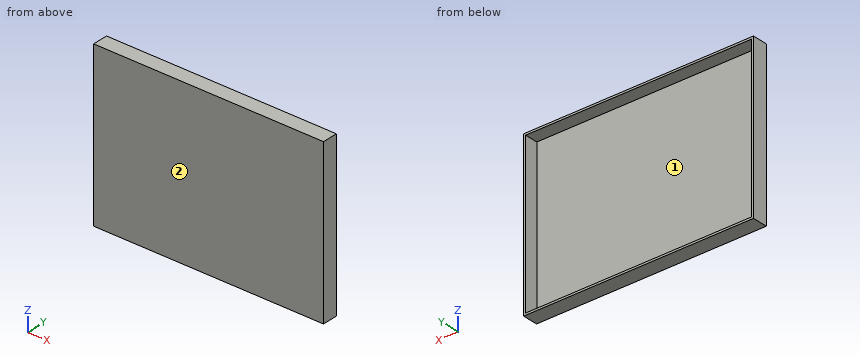
```python
from build123d import *

# Parameters (mm, degrees)
SKETCH1_W           = 343
SKETCH1_H           = 243
SKETCH1_W_2         = 337
SKETCH1_H_2         = 237
BOSS_EXTRUDE1_DEPTH = 23
SKETCH2_W           = 343
SKETCH2_H           = 243
BOSS_EXTRUDE2_DEPTH = 3


with BuildPart() as part:
    # Sketch1 → Boss-Extrude1 (new body)
    with BuildSketch(Plane(origin=(0, 0, 0), x_dir=(1, 0, 0), z_dir=(0, 1, 0))):
        Rectangle(SKETCH1_W, SKETCH1_H)
        Rectangle(SKETCH1_W_2, SKETCH1_H_2, mode=Mode.SUBTRACT)
    extrude(amount=BOSS_EXTRUDE1_DEPTH)

    # Sketch2 → Boss-Extrude2 (add)
    with BuildSketch(Plane.XZ):
        Rectangle(SKETCH2_W, SKETCH2_H)
    extrude(amount=-BOSS_EXTRUDE2_DEPTH)


solid = part.part
```
For this review, take the finished solid that the model builds, in its own axes (mm). Face numbers are marked on the shaded views. Round coordinates to 2 decimals unless told otherwise and drop trailing zeros. Write each loop counter-clockwise with the first axis right and the second up, starting at its lowest first coordinate (ties: lowest second). Pieces come first, ordered by that corner, then holes. Notation, with made-up numbers: (47.25, 3.5) - (71.25, 3.5) arc R37 ccw to (71.25, 39.5) - close; hole circle Ø9 at (83, 62.5). An arc over 180 degrees is marked (long way). Put each result on its own line as item: value.
Q1. We need section C-C (x = 134). Give the boundary of the cut face in (y, z).
Solved:
outline: (0, -121.5) - (23, -121.5) - (23, -118.5) - (3, -118.5) - (3, 118.5) - (23, 118.5) - (23, 121.5) - (0, 121.5) - close
Q2. We need section A-A (y = 19). Give the boundary of the cut face in (x, z).
Solved:
outline: (-171.5, -121.5) - (171.5, -121.5) - (171.5, 121.5) - (-171.5, 121.5) - close; hole (-168.5, -118.5) - (168.5, -118.5) - (168.5, 118.5) - (-168.5, 118.5) - close
Q3. Wall thickness on probe 1 along Z at (x, y) = (-6, 14.75); probe 2 along X at (y, z) = (20, 42.5); probe 3 along Y at (x, z) = (-58, 56): over which ranges is each line inside the solid? List them lowest first.
Solved:
probe 1: z = -121.5 to -118.5, 118.5 to 121.5
probe 2: x = -171.5 to -168.5, 168.5 to 171.5
probe 3: y = 0 to 3
Q4. Mouldability with a two-part tool opening along Z and no side actions: class the marked faces 1 and 2 as released by +Z, released by -Z, zero draft, split by the parting line, or undercut.
Solved:
face 1: undercut
face 2: zero draft
Q5. We need section B-B (z = -23.5). Give the boundary of the cut face in (x, y), and give its area (3 significant figures).
Solved:
outline: (-171.5, 0) - (171.5, 0) - (171.5, 23) - (168.5, 23) - (168.5, 3) - (-168.5, 3) - (-168.5, 23) - (-171.5, 23) - close
area: 1,150 mm2
